Geometry check sheet. Reference: the model listing, model coordinates, mm. A direction names the side the tool comes from. Give positions to 0.01 mm unless a question says otherwise; leave off trailing zeros. Order: outer loops, then holes, each group sorted by start corner. A loop starts at its lowest first (then second) coordinate and runs counter-clockwise, first axis right, second up. Notation, with made-up numbers: M 5,40.5 L 59,40.5 A36 ccw 59,74.5 Z; hole C 41.25,53.5 d10. An arc over 180 degrees is marked long. Answer as CSV lines item,"result". Start each with the question number.
```python
from build123d import *

# Parameters (mm, degrees)
ESQUISSE1_R              = 5
ESQUISSE1_R_2            = 2.25
BOSS_EXTRU_1_DEPTH       = 4
CONG_2_R                 = 6
CONG_3_R                 = 20
ESQUISSE4_R              = 12.75
ENL_V_MAT_EXTRU_20_DEPTH = 1.5


with BuildPart() as part:
    # Esquisse1 → Boss.-Extru.1 (new body)
    with BuildSketch(Plane.XY):
        Polygon((-55, 20), (-27.5, 0), (0, 20), (0, 40), (-55, 40), align=None)
        with Locations((-27.5, 27.5)):
            Circle(ESQUISSE1_R, mode=Mode.SUBTRACT)
        with Locations((-47.5, 32.5)):
            Circle(ESQUISSE1_R_2, mode=Mode.SUBTRACT)
        with Locations((-7.5, 32.5)):
            Circle(ESQUISSE1_R_2, mode=Mode.SUBTRACT)
        with Locations((-27.5, 7.5)):
            Circle(ESQUISSE1_R_2, mode=Mode.SUBTRACT)
    extrude(amount=BOSS_EXTRU_1_DEPTH)

    # Congé2
    cong_2_edges = [part.edges().sort_by_distance(p)[0] for p in [
        (-55, 40, 2),
        (0, 40, 2),
        (-27.5, 0, 2),
    ]]
    fillet(cong_2_edges, radius=CONG_2_R)

    # Congé3
    cong_3_edges = [part.edges().sort_by_distance(p)[0] for p in [
        (0, 20, 2),
        (-55, 20, 2),
    ]]
    fillet(cong_3_edges, radius=CONG_3_R)

    # Esquisse4 → Enlèv. mat.-Extru.20 (cut)
    with BuildSketch(Plane(origin=(0, 0, 0), x_dir=(-1, 0, 0), z_dir=(0, 0, -1))):
        with Locations((27.5, 27.5)):
            Circle(ESQUISSE4_R)
    extrude(amount=-ENL_V_MAT_EXTRU_20_DEPTH, mode=Mode.SUBTRACT)


solid = part.part
```
Item 1: Draft check along Y on faces 3 (the face through (-2.24, 20.99, 2.03)), 4 (the face through (0, 32, 2)), 5 (the face through (-25.354, 8.176, 1.972)). Enter one of: pulls with the +Y half, pulls with the -Y half, needs draft (parallel to the pull), parting line crosses it, or undercut.
Item 2: Section check D-D on x = -19. Record the boundary of the cut face in (y, z), then the cut area to 3 significant figures.
Item 3: Section check B-B on y = 7.5. Record the boundary of the cut face in (x, z).
Item 4: Depth check by flat-ended pin: pin 1 Ø3 at (x, y) = (-35, 30.5) entering from -Z; pin 2 Ø1 at (x, z) = (-45, 3) entering from -Y; pin 3 Ø1.5 at (y, z) = (15.5, 1) entering from +X. Enter the tip coordinate at first touch or a pass-through.
Item 5: Scan lines: line 1 along Z through (x, y) = (-29.5, 37); line 2 along Y through (x, z) = (-33, 1.2); line 3 along X through (y, z) = (14, 3.15). Record each from-to range of solid material in increasing order.
Item 6: Access from +Z, -Z, +X, -X, +Y, -Y to the whole of each face (thin tool, end or side, straight path). Record for faces 1 (the face through (-26.97, 14.76, 0.74)), 2 (the face through (-55, 32, 2)).
Item 7: Section check C-C on x = -47.5. Record the boundary of the cut face in (y, z), then the cut area to 3 significant figures.
Item 8: Section check A-A on z = 2.45. Record the boundary of the cut face in (x, y), then the cut area to 3 significant figures.
Numbers:
1,face 3,"pulls with the -Y half"
1,face 4,"needs draft"
1,face 5,"undercut"
2,outline,"M 6.18,0 L 18,0 L 18,1.5 L 37,1.5 L 37,0 L 40,0 L 40,4 L 6.18,4 Z"
2,area,"107 mm2"
3,outline,"M -37.81,0 L -29.75,0 L -29.75,4 L -37.81,4 Z; M -25.25,0 L -17.19,0 L -17.19,4 L -25.25,4 Z"
4,pin 1,"z = 1.5"
4,pin 2,"y = 12.36"
4,pin 3,"x = -5.65"
5,line 1,"1.5 to 4"
5,line 2,"4 to 16, 39 to 40"
5,line 3,"-46.75 to -8.25"
6,face 1,"-Z"
6,face 2,"+Z, -Z, -X, +Y, -Y"
7,outline,"M 14.57,0 L 30.25,0 L 30.25,4 L 14.57,4 Z; M 34.75,0 L 40,0 L 40,4 L 34.75,4 Z"
7,area,"83.7 mm2"
8,outline,"M -55,30.18 A20 ccw -46.76,14.01 L -31.03,2.57 A6 ccw -23.97,2.57 L -8.24,14.01 A20 ccw 0,30.18 L 0,34 A6 ccw -6,40 L -49,40 A6 ccw -55,34 Z; hole C -47.5,32.5 d4.5; hole C -27.5,27.5 d10; hole C -27.5,7.5 d4.5; hole C -7.5,32.5 d4.5"
8,area,"1,470 mm2"
